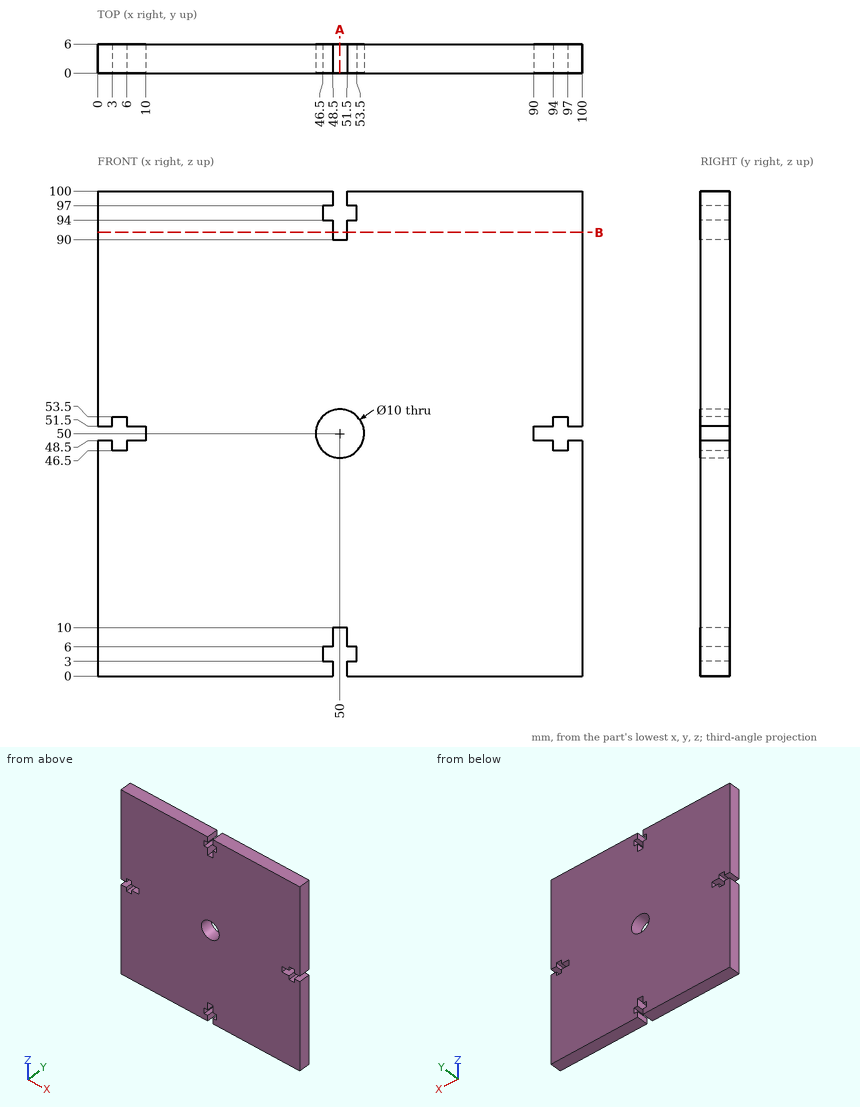
Part print with two shaded views. Sizes in mm from the minimum x, y, z corner. Give positions to 0.01 mm unless a question says otherwise; leave off trailing zeros. Order: outer loops, then holes, each group sorted by start corner. A loop starts at its lowest first (then second) coordinate and runs counter-clockwise, first axis right, second up.
(1) Saw through at B-B, the plane z = 91.5. Give the cut face in (x, y).
(2) Saw through at A-A, the plane x = 50. Give the cut face in (y, z), then the cut area to 3 significant figures.
(3) Flat gauge pins, fed straight in: pin 1 (0.9 mm diameter, centred on x = 50.5, y = 2.5, fed in from -Z); pin 2 (1.5 mm diameter, centred on y = 3, z = 50.5, fed in from +X). Where does each tip first touch, or does it go through?
(4) Drill centre lines: L1, parallel to X at y = 2.55, z = 50; L2, parallel to Z at x = 9, y = 3; L3, parallel to Z at x = 49, y = 1.35. Where is each one in solid material? Low to high.
Results found:
1. outline: (0, 0) - (48.5, 0) - (48.5, 6) - (0, 6) - close; (51.5, 0) - (100, 0) - (100, 6) - (51.5, 6) - close
2. outline: (0, 10) - (6, 10) - (6, 45) - (0, 45) - close; (0, 55) - (6, 55) - (6, 90) - (0, 90) - close
2. area: 420 mm2
3. pin 1: stops at z = 10
3. pin 2: stops at x = 90
4. L1: x = 10 to 45, 55 to 90
4. L2: z = 0 to 48.5, 51.5 to 100
4. L3: z = 10 to 45.1, 54.9 to 90
